Could you check a few things on this model? Use its own coordinates, in mm. Coordinates: 2 decimals unless noted, no trailing zeros. Loops run counter-clockwise (first coordinate to the right, second up) from the corner with the lowest first, then second, coordinate; pieces in that order, holes last.
1) Imagine slicing it at A-A on x = 50.8. Please give me the cut outline in (y, z), plus the area to 3 significant figures.
2) If I drill on line 1 along Z through (x, y) = (50.8, -8); line 2 along Z through (x, y) = (54, -3.75); line 3 along X through (y, z) = (-4.5, 4), over which ranges is the centre line in solid material (lowest first)?
3) Will this pin go through, and if not, where does the flat tip stop? P1, Ø4, axis at x = 58.5, z = 70.5, coming from the +Y side.
4) Imagine slicing it at B-B on z = 50.8. Please give me the cut outline in (x, y), plus the area to 3 significant figures.
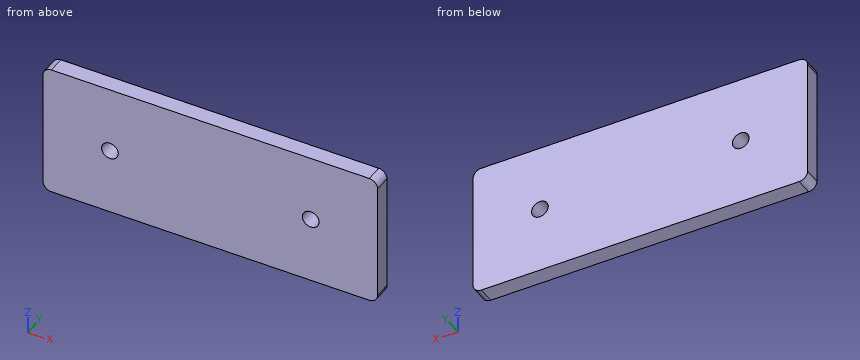
```python
from build123d import *

# Parameters (mm, degrees)
F0_W     = 254
F0_H     = 101.6
F0_R     = 6.35
F1_DEPTH = 12.7
F2_R     = 6.35


with BuildPart() as f1:
    # F0 (on Front) → F1 (new body)
    with BuildSketch(Plane.XZ):
        with Locations((127, 50.8)):
            Rectangle(F0_W, F0_H)
        with Locations((50.8, 50.8)):
            Circle(F0_R, mode=Mode.SUBTRACT)
        with Locations((203.2, 50.8)):
            Circle(F0_R, mode=Mode.SUBTRACT)
    extrude(amount=F1_DEPTH)

    # F2
    f2_edges = [f1.edges().sort_by_distance(p)[0] for p in [
        (0, -6.35, 101.6),
        (254, -6.35, 101.6),
        (254, -6.35, 0),
        (0, -6.35, 0),
    ]]
    fillet(f2_edges, radius=F2_R)


solid = f1.part
```
Filled in:
1. outline: (-12.7, 0) - (0, 0) - (0, 44.45) - (-12.7, 44.45) - close; (-12.7, 57.15) - (0, 57.15) - (0, 101.6) - (-12.7, 101.6) - close
1. area: 1,130 mm2
2. line 1: z = 0 to 44.45, 57.15 to 101.6
2. line 2: z = 0 to 45.32, 56.28 to 101.6
2. line 3: x = 0.45 to 253.55
3. P1: stops at y = 0
4. outline: (0, -12.7) - (44.45, -12.7) - (44.45, 0) - (0, 0) - close; (57.15, -12.7) - (196.85, -12.7) - (196.85, 0) - (57.15, 0) - close; (209.55, -12.7) - (254, -12.7) - (254, 0) - (209.55, 0) - close
4. area: 2,900 mm2
